Print and shaded views of the part. All mm, measured from the part's lowest x, y and z. Round coordinates to 2 decimals unless told otherwise and drop trailing zeros. Order: outer loops, then holes, each group sorted by start corner. A loop starts at its lowest first (then second) coordinate and runs counter-clockwise, first axis right, second up. Notation, with made-up numbers: (65, 22) - (86, 22) arc R26 ccw to (86, 38) - close; hole circle Ø8 at (39.5, 18). An arc over 180 degrees is marked (long way). Return JSON: item names as keys, results as strings. Group by question number.
Item 1: Probe probe 1 along Y at (x, z) = (3, 5); probe 2 along X at (y, z) = (3.5, 4.25); probe 3 along Y at (x, z) = (2, 1). List the from-to ranges inside material, lowest first.
Item 2: Saw through at A-A on z = 4.75. List the corners of the cut face in (x, y).
Item 3: Saw through at B-B on x = 6.75. List the corners of the cut face in (y, z).
Item 4: Drop flat-ended pins along their axis: pin 1 (1.5 mm diameter, centred on x = 6, z = 4.5, fed in from -Y); pin 2 (1 mm diameter, centred on y = 4, z = 2.5, fed in from +X). Give the stop position or say it passes through.
Item 5: Two-plate mould, pull along Y, no slides. Class the marked faces 1, 2 and 3: released by +Y, released by -Y, zero draft, split by the parting line, or undercut.
Item 6: Saw through at C-C on y = 5.25. List the corners of the cut face in (x, z).
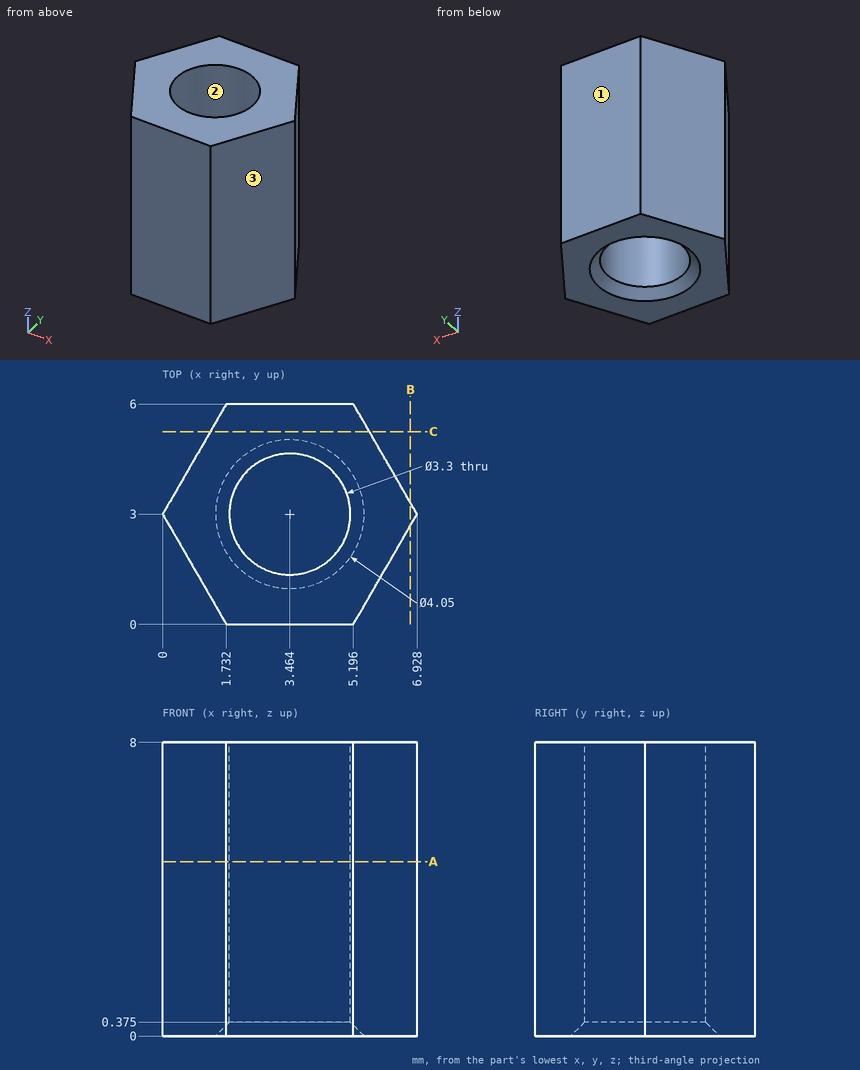
Filled in:
{
 "1": {"probe 1": "y = 0 to 1.42, 4.58 to 6", "probe 2": "x = 0.29 to 1.89, 5.04 to 6.64", "probe 3": "y = 0 to 2.24, 3.76 to 6"},
 "2": {"outline": "(0, 3) - (1.73, 0) - (5.2, 0) - (6.93, 3) - (5.2, 6) - (1.73, 6) - close; hole circle Ø3.3 at (3.46, 3)"},
 "3": {"outline": "(2.69, 0) - (3.31, 0) - (3.31, 8) - (2.69, 8) - close"},
 "4": {"pin 1": "stops at y = 0.09", "pin 2": "stops at x = 6.64"},
 "5": {"face 1": "released by +Y", "face 2": "undercut", "face 3": "released by -Y"},
 "6": {"outline": "(1.3, 0) - (5.63, 0) - (5.63, 8) - (1.3, 8) - close"}
}
